from build123d import *

# Parameters (mm, degrees)
SKETCH1_W           = 304.8
SKETCH1_H           = 304.8
SKETCH1_R           = 2.5527
SKETCH1_R_2         = 2.54
SKETCH1_R_3         = 3.2639
BOSS_EXTRUDE1_DEPTH = 3.175


with BuildPart() as part:
    # Sketch1 → Boss-Extrude1 (new body)
    with BuildSketch(Plane.XY):
        Rectangle(SKETCH1_W, SKETCH1_H)
        with Locations((-76.2, 127)):
            Circle(SKETCH1_R, mode=Mode.SUBTRACT)
        with Locations((-25.4, 127)):
            Circle(SKETCH1_R, mode=Mode.SUBTRACT)
        with Locations((25.4, 127)):
            Circle(SKETCH1_R, mode=Mode.SUBTRACT)
        with Locations((76.2, 127)):
            Circle(SKETCH1_R, mode=Mode.SUBTRACT)
        with Locations((-101.6, 0)):
            Circle(SKETCH1_R_2, mode=Mode.SUBTRACT)
        with Locations((-50.8, 0)):
            Circle(SKETCH1_R_2, mode=Mode.SUBTRACT)
        Circle(SKETCH1_R_2, mode=Mode.SUBTRACT)
        with Locations((101.6, 0)):
            Circle(SKETCH1_R_2, mode=Mode.SUBTRACT)
        with Locations((50.8, 0)):
            Circle(SKETCH1_R_2, mode=Mode.SUBTRACT)
        with Locations((-50.8, 127)):
            Circle(SKETCH1_R_2, mode=Mode.SUBTRACT)
        with Locations((0, 127)):
            Circle(SKETCH1_R_2, mode=Mode.SUBTRACT)
        with Locations((50.8, 127)):
            Circle(SKETCH1_R_2, mode=Mode.SUBTRACT)
        with Locations((-101.6, 72.39)):
            Circle(SKETCH1_R_2, mode=Mode.SUBTRACT)
        with Locations((0, 72.39)):
            Circle(SKETCH1_R_2, mode=Mode.SUBTRACT)
        with Locations((101.6, 72.39)):
            Circle(SKETCH1_R_2, mode=Mode.SUBTRACT)
        with Locations((-101.6, -72.39)):
            Circle(SKETCH1_R_2, mode=Mode.SUBTRACT)
        with Locations((0, -72.39)):
            Circle(SKETCH1_R_2, mode=Mode.SUBTRACT)
        with Locations((101.6, -72.39)):
            Circle(SKETCH1_R_2, mode=Mode.SUBTRACT)
        with Locations((-76.2, -127)):
            Circle(SKETCH1_R, mode=Mode.SUBTRACT)
        with Locations((-25.4, -127)):
            Circle(SKETCH1_R, mode=Mode.SUBTRACT)
        with Locations((25.4, -127)):
            Circle(SKETCH1_R, mode=Mode.SUBTRACT)
        with Locations((76.2, -127)):
            Circle(SKETCH1_R, mode=Mode.SUBTRACT)
        with Locations((50.8, -127)):
            Circle(SKETCH1_R_2, mode=Mode.SUBTRACT)
        with Locations((0, -127)):
            Circle(SKETCH1_R_2, mode=Mode.SUBTRACT)
        with Locations((-50.8, -127)):
            Circle(SKETCH1_R_2, mode=Mode.SUBTRACT)
        with Locations((-101.6, 97.79)):
            Circle(SKETCH1_R_2, mode=Mode.SUBTRACT)
        with Locations((0, 97.79)):
            Circle(SKETCH1_R_2, mode=Mode.SUBTRACT)
        with Locations((101.6, 97.79)):
            Circle(SKETCH1_R_2, mode=Mode.SUBTRACT)
        with Locations((101.6, 127)):
            Circle(SKETCH1_R_2, mode=Mode.SUBTRACT)
        with Locations((-101.6, 127)):
            Circle(SKETCH1_R_2, mode=Mode.SUBTRACT)
        with Locations((-118.11, 33.02)):
            Circle(SKETCH1_R_2, mode=Mode.SUBTRACT)
        with Locations((-101.6, -127)):
            Circle(SKETCH1_R_2, mode=Mode.SUBTRACT)
        with Locations((101.6, -127)):
            Circle(SKETCH1_R_2, mode=Mode.SUBTRACT)
        with Locations((101.6, -97.79)):
            Circle(SKETCH1_R_2, mode=Mode.SUBTRACT)
        with Locations((0, -97.79)):
            Circle(SKETCH1_R_2, mode=Mode.SUBTRACT)
        with Locations((-101.6, -97.79)):
            Circle(SKETCH1_R_2, mode=Mode.SUBTRACT)
        with Locations((-118.11, -33.02)):
            Circle(SKETCH1_R_2, mode=Mode.SUBTRACT)
        with Locations((-139.7, 139.7)):
            Circle(SKETCH1_R_3, mode=Mode.SUBTRACT)
        with Locations((-139.7, 0)):
            Circle(SKETCH1_R_3, mode=Mode.SUBTRACT)
        with Locations((-139.7, -139.7)):
            Circle(SKETCH1_R_3, mode=Mode.SUBTRACT)
        with Locations((139.7, -139.7)):
            Circle(SKETCH1_R_3, mode=Mode.SUBTRACT)
        with Locations((139.7, 0)):
            Circle(SKETCH1_R_3, mode=Mode.SUBTRACT)
        with Locations((139.7, 139.7)):
            Circle(SKETCH1_R_3, mode=Mode.SUBTRACT)
        with Locations((118.11, -33.02)):
            Circle(SKETCH1_R_2, mode=Mode.SUBTRACT)
        with Locations((118.11, 33.02)):
            Circle(SKETCH1_R_2, mode=Mode.SUBTRACT)
    extrude(amount=BOSS_EXTRUDE1_DEPTH)


solid = part.part
Source: CAD feature listing. Evaluate the final solid. Frame: model axes, mm. Coordinates: 2 decimals unless noted, no trailing zeros. Write each question's results on one line, items separated by ' | '. Start each with the question number.
Item 1: Line query: probe 1 along Y at (x, z) = (-50.8, 1.15); probe 2 along Y at (x, z) = (-25.4, 0.8); probe 3 along X at (y, z) = (139.7, 0.75). Output: solid intervals per line, ascending.
Item 2: First-contact query: pin 1 Ø4.5 at (x, y) = (-76.2, 127) entering from -Z. Flat tip, straight axial feed; report the tip coordinate or a pass-through.
Item 3: Draft query along Y for faces 1 (the face through (-2, 2, 3.175)), 2 (the face through (142.715, -1.25, 1.565)). Return one class per face: pulls with the +Y half, pulls with the -Y half, needs draft (parallel to the pull), parting line crosses it, or undercut.
Checked values:
1) probe 1: y = -152.4 to -129.54, -124.46 to -2.54, 2.54 to 124.46, 129.54 to 152.4 | probe 2: y = -152.4 to -129.55, -124.45 to 124.45, 129.55 to 152.4 | probe 3: x = -152.4 to -142.96, -136.44 to 136.44, 142.96 to 152.4
2) pin 1: passes through
3) face 1: needs draft | face 2: undercut
